Here's the drawing with two shaded views (mm, measured from the low corner). I have some questions. Round coordinates to 2 decimals unless told otherwise and drop trailing zeros. Loops run counter-clockwise (first coordinate to the right, second up) from the corner with the lowest first, then second, coordinate; pieces in that order, holes last.
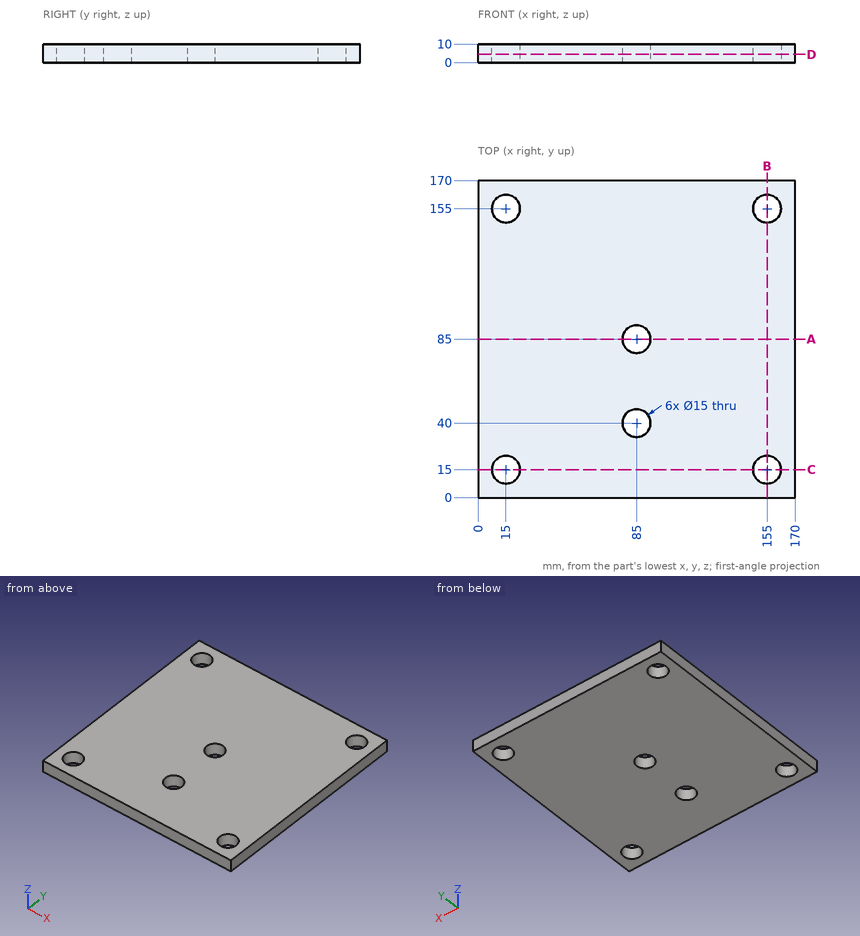
Item 1: Will this pin go through, and if not, where does the flat tip stop? pin 1 (12 mm diameter, centred on x = 155, y = 15, fed in from +Z).
Results list:
pin 1: passes through
Item 2: If we section it at A-A, the plane y = 85: Please give me the cut outline in (x, z), then the cut area to 3 significant figures.
Results list:
outline: (0, 0) - (77.5, 0) - (77.5, 10) - (0, 10) - close; (92.5, 0) - (170, 0) - (170, 10) - (92.5, 10) - close
area: 1,550 mm2
Item 3: If we section it at B-B, the plane x = 155: Please give me the cut outline in (y, z).
Results list:
outline: (0, 0) - (7.5, 0) - (7.5, 10) - (0, 10) - close; (22.5, 0) - (147.5, 0) - (147.5, 10) - (22.5, 10) - close; (162.5, 0) - (170, 0) - (170, 10) - (162.5, 10) - close
Item 4: If I drill on line 1 along X through (y, z) = (15, 3); line 2 along Y through (x, z) = (85, 6.5), over which ranges is the centre line in solid material (lowest first)?
Results list:
line 1: x = 0 to 7.5, 22.5 to 147.5, 162.5 to 170
line 2: y = 0 to 32.5, 47.5 to 77.5, 92.5 to 170
Item 5: If we section it at D-D, the plane z = 4.5: Please give me the cut outline in (x, y).
Results list:
outline: (0, 0) - (170, 0) - (170, 170) - (0, 170) - close; hole circle Ø15 at (15, 15); hole circle Ø15 at (15, 155); hole circle Ø15 at (85, 40); hole circle Ø15 at (85, 85); hole circle Ø15 at (155, 15); hole circle Ø15 at (155, 155)
